Could you check a few things on this model? Use its own coordinates, in mm. Face numbers are marked on the shaded views. Round coordinates to 2 decimals unless told otherwise and drop trailing zeros. Loops run counter-clockwise (first coordinate to the right, second up) from the corner with the lowest first, then second, coordinate; pieces in that order, holes last. Notation, with made-up numbers: (-19, 32.25) -> (-11, 32.25) arc R23 ccw to (-11, 49.25) -> close; hole circle Ø10 at (28.25, 51). An arc over 180 degrees is marked (long way). One line per item, written item: value.
from build123d import *

# Parameters (mm, degrees)
F0_R        = 12.3317
F0_R_2      = 11.176
F1_DEPTH    = 47.5
F0_R_3      = 8.89
F2_DEPTH    = 40.5
F3_S5_R     = 11.176
F3_T6_DEPTH = 18


# Not quite as in the source:
# - a fillet or chamfer that OpenCascade refuses, or shapes differently, is made with other operations: its cross-section is extruded or revolved along the edge and cut away or added


with BuildPart() as f1:
    # F0 (on Top) → F1 (new body, symmetric)
    with BuildSketch(Plane.XY):
        Circle(F0_R)
        Circle(F0_R_2, mode=Mode.SUBTRACT)
    extrude(amount=F1_DEPTH, both=True)

    # F0 (on Top) → F2 (join, symmetric)
    with BuildSketch(Plane.XY):
        Circle(F0_R_2)
        Circle(F0_R_3, mode=Mode.SUBTRACT)
    extrude(amount=F2_DEPTH, both=True)

    # F3: chamfer of 2.54 on 1 edges, made by hand


with BuildPart() as f3_tool2:
    # F3_s3 → F3_t4 (revolve)
    with BuildSketch(Plane.XZ):
        Polygon((11.43, -40.5), (8.89, -37.96), (8.89, -40.5), align=None)
    revolve(axis=Axis((0, 0, -40.5), (0, 0, 1)))

    # F3_s5 → F3_t6 (intersect, symmetric)
    with BuildSketch(Plane.XY.offset(-39.2)):
        Circle(F3_S5_R)
    extrude(amount=F3_T6_DEPTH, both=True, mode=Mode.INTERSECT)


with BuildPart() as f1_1:
    add(f1.part)

    # F3_t1: cut F3_tool2
    add(f3_tool2.part, mode=Mode.SUBTRACT)


solid = f1_1.part
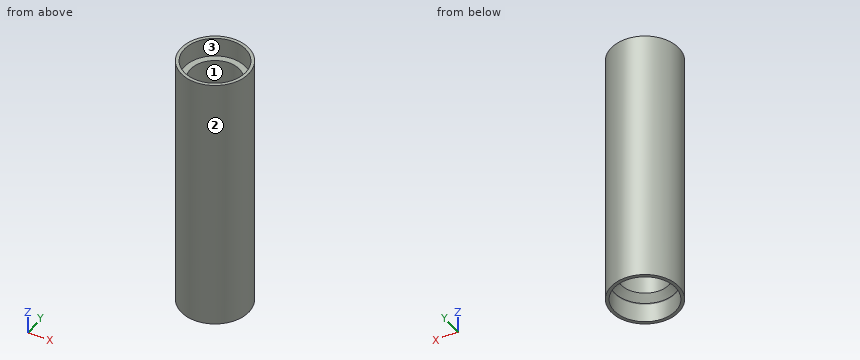
(1) If we section it at A-A, the plane y = 0: Please give me the cut outline in (x, z), then the cut area to 3 significant figures.
Recorded:
outline: (-12.33, -47.5) -> (-11.18, -47.5) -> (-11.18, -40.25) -> (-8.89, -37.96) -> (-8.89, 40.5) -> (-11.18, 40.5) -> (-11.18, 47.5) -> (-12.33, 47.5) -> close; (8.89, -37.96) -> (11.18, -40.25) -> (11.18, -47.5) -> (12.33, -47.5) -> (12.33, 47.5) -> (11.18, 47.5) -> (11.18, 40.5) -> (8.89, 40.5) -> close
area: 584 mm²
(2) I'm going to push flat-ended pins straight in: pin 1 Ø14 at (x, y) = (0, 0) entering from +Z; pin 2 Ø4 at (x, z) = (8, -13.5) entering from +Y; pin 3 Ø4 at (y, z) = (-4.5, 32.5) entering from -X; pin 4 Ø5 at (x, y) = (-6, 5) entering from +Z. Where does each tip first touch, or does it pass through?
Recorded:
pin 1: through
pin 2: y = 10.77
pin 3: x = -12.08
pin 4: z = 40.5
(3) Thinking about a two-plate mould opening in Y: for the marked faces 1, 2 and 3, which applies, released by +Y, released by -Y, zero draft, split by the parting line, or undercut?
Recorded:
face 1: undercut
face 2: split by the parting line
face 3: undercut
(4) If I drill on L1, parallel to Y at x = 0, z = 43.5; L2, parallel to Y at x = 0, z = 11.5; L3, parallel to X at y = -1.25, z = -9.5, over which ranges is the centre line in solid material (lowest first)?
Recorded:
L1: -12.33 to -11.18, 11.18 to 12.33
L2: -12.33 to -8.89, 8.89 to 12.33
L3: -12.27 to -8.8, 8.8 to 12.27
(5) If we section it at C-C, the plane z = 19.5: Please give me the cut outline in (x, y), then the cut area to 3 significant figures.
Recorded:
outline: circle Ø24.66 at (0, 0); hole circle Ø17.78 at (0, 0)
area: 229 mm²
